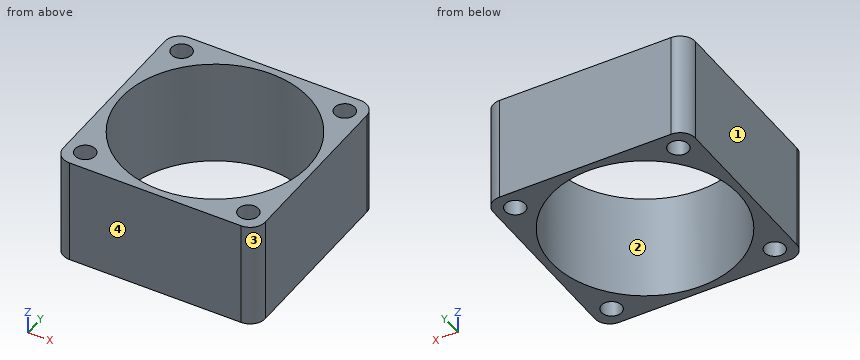
Autodesk Fusion 360 part; units mm, degrees
box "BoxPrimitive1" add length 40 width 40 height 21 placed x (0, -1, 0) y (1, 0, 0) z (0, 0, 1) at (40, 0, 0)
fillet "Fillet1" radius 3 4 edges at (40, -40, 10.5) (80, -40, 10.5) (80, 0, 10.5) (40, 0, 10.5)
sketch "Sketch2" plane through (0, 0, 21) normal (0, 0, 1) x (-1, 0, 0)
  arc A0 (-43, 0) -> (-40, 3) centre (-43, 3) ccw
  line L0 (-40, 3) -> (-40, 37)
  arc A1 (-40, 37) -> (-43, 40) centre (-43, 37) ccw
  line L1 (-43, 40) -> (-77, 40)
  arc A2 (-77, 40) -> (-80, 37) centre (-77, 37) ccw
  line L2 (-80, 37) -> (-80, 3)
  arc A3 (-80, 3) -> (-77, 0) centre (-77, 3) ccw
  line L3 (-77, 0) -> (-43, 0)
  circle A4 centre (-76.15, 36.15) radius 2
  circle A5 centre (-76.15, 3.85) radius 2
  circle A6 centre (-43.85, 36.15) radius 2
  circle A7 centre (-43.85, 3.85) radius 2
  line L4 (-40.8787, 0.8787) -> (-79.1213, 39.1213) construction
  line L5 (-40.8787, 39.1213) -> (-79.1213, 0.8787) construction
  circle A8 centre (-60, 20) radius 18.55
  dimension "d8" = 4
  dimension "d9" = 4
  dimension "d10" = 4
  dimension "d11" = 4
  dimension "d12" = 3.85
  dimension "d13" = 3.85
  dimension "d14" = 3.85
  dimension "d15" = 3.85
  dimension "d16" = 3.85
  dimension "d17" = 3.85
  dimension "d18" = 3.85
  dimension "d19" = 3.85
  dimension "d23" = 37.1
extrude "Extrude1" cut sketch "Sketch2" against normal blind 35 contours A4 | A5 | A6 | A7
extrude "Extrude2" cut sketch "Sketch2" against normal blind 35 contours A8
equation "d12 = screw_spacing"
equation "d13 = screw_spacing"
equation "d14 = screw_spacing"
equation "d15 = screw_spacing"
equation "d16 = screw_spacing"
equation "d17 = screw_spacing"
equation "d18 = screw_spacing"
equation "d19 = screw_spacing"
equation "screw_spacing = 3.85 mm"
Verification items for the finished model (mm, model axes). Face numbers are marked on the shaded views. Give positions to 0.01 mm unless a question says otherwise; leave off trailing zeros. Write each loop counter-clockwise with the first axis right and the second up, starting at its lowest first coordinate (ties: lowest second). Pieces come first, ordered by that corner, then holes. Notation, with made-up numbers: (-27, -25.5) -> (12, -25.5) arc R8 cw to (12, -17.5) -> close; hole circle Ø4 at (35.25, 89.5). An arc over 180 degrees is marked (long way). Use CSV: the item, a comma, the result in double quotes.
(1) Sectioned sample at A-A (x = 60). Record the cut outline in (y, z), plus the area to 3 significant figures.
Derived:
outline,"(-40, 0) -> (-38.55, 0) -> (-38.55, 21) -> (-40, 21) -> close; (-1.45, 0) -> (0, 0) -> (0, 21) -> (-1.45, 21) -> close"
area,"60.9 mm^2"
(2) Sectioned sample at D-D (x = 76). Record the cut outline in (y, z).
Derived:
outline,"(-40, 0) -> (-38.14, 0) -> (-38.14, 21) -> (-40, 21) -> close; (-34.16, 0) -> (-29.39, 0) -> (-29.39, 21) -> (-34.16, 21) -> close; (-10.61, 0) -> (-5.84, 0) -> (-5.84, 21) -> (-10.61, 21) -> close; (-1.86, 0) -> (0, 0) -> (0, 21) -> (-1.86, 21) -> close"
(3) Sectioned sample at C-C (y = -36.15). Record the cut outline in (x, z).
Derived:
outline,"(40, 0) -> (41.85, 0) -> (41.85, 21) -> (40, 21) -> close; (45.85, 0) -> (50.87, 0) -> (50.87, 21) -> (45.85, 21) -> close; (69.13, 0) -> (74.15, 0) -> (74.15, 21) -> (69.13, 21) -> close; (78.15, 0) -> (80, 0) -> (80, 21) -> (78.15, 21) -> close"
(4) Sectioned sample at B-B (y = -20). Record the cut outline in (x, z), plus the area to 3 significant figures.
Derived:
outline,"(40, 0) -> (41.45, 0) -> (41.45, 21) -> (40, 21) -> close; (78.55, 0) -> (80, 0) -> (80, 21) -> (78.55, 21) -> close"
area,"60.9 mm^2"
(5) Material ranges on L1, parallel to Y at x = 43.85, z = 7; L2, parallel to X at y = -32, z = 15.25; L3, parallel to Y at x = 60, z = 10, recorded low to high.
Derived:
L1,"y = -40 to -38.15, -34.15 to -29.13, -10.87 to -5.85, -1.85 to 0"
L2,"x = 40 to 45.85, 74.15 to 80"
L3,"y = -40 to -38.55, -1.45 to 0"
(6) Release check for a two-part mould opening along X. For the marked faces 1, 2, 3 and 4 record: +X half, -X half, draft (parallel to the pull), parting line (faces both ways), or undercut.
Derived:
face 1,"-X half"
face 2,"undercut"
face 3,"+X half"
face 4,"draft"
